from build123d import *

# Parameters (mm, degrees)
BOSS_EXTRUDE3_DEPTH = 31.75
BOSS_EXTRUDE4_DEPTH = 25.4
SKETCH3_R           = 12.7
BOSS_EXTRUDE5_DEPTH = 76.2


with BuildPart() as part:
    # Sketch1 → Boss-Extrude3 (new body)
    with BuildSketch(Plane.XY):
        with BuildLine():
            Line((-30.208002872, 9.539170605), (-46.704713672, 0.008989394))
            Line((-46.704713672, 0.008989394), (-30.209378213, -9.523572129))
            ThreePointArc((-30.209378213, -9.523572129), (-28.303227656, -4.925697376), (-27.653051773, 0.008989394))
            ThreePointArc((-27.653051773, 0.008989394), (-28.302871676, 4.942348519), (-30.208002872, 9.539170605))
        make_face()
        with BuildLine():
            Line((-30.209378213, -9.523572129), (-46.704713672, 0.008989394))
            Line((-46.704713672, 0.008989394), (-30.208002872, 9.539170605))
            ThreePointArc((-30.208002872, 9.539170605), (-65.756375522, 0.010363935), (-30.209378213, -9.523572129))
        make_face()
        with BuildLine():
            ThreePointArc((65.756375572, 53.972753345), (41.773446789, 72.372990127), (30.211103799, 44.443403463))
            Line((30.211103799, 44.443403463), (46.706375572, 53.972753345))
            Line((46.706375572, 53.972753345), (46.706375572, 34.922753345))
            ThreePointArc((46.706375572, 34.922753345), (60.176759753, 40.502369163), (65.756375572, 53.972753345))
        make_face()
        with BuildLine():
            Line((46.706375572, 53.972753345), (30.211103799, 44.443403463))
            ThreePointArc((30.211103799, 44.443403463), (37.183550761, 37.473713748), (46.706375572, 34.922753345))
            Line((46.706375572, 34.922753345), (46.706375572, 53.972753345))
        make_face()
        with BuildLine():
            ThreePointArc((46.706375572, -34.922753345), (37.184741159, -37.473026737), (30.21247902, -44.441023358))
            Line((30.21247902, -44.441023358), (46.706375572, -53.972753345))
            Line((46.706375572, -53.972753345), (46.706375572, -34.922753345))
        make_face()
        with BuildLine():
            Line((46.706375572, -53.972753345), (30.21247902, -44.441023358))
            ThreePointArc((30.21247902, -44.441023358), (41.772119261, -72.372634177), (65.756375572, -53.972753345))
            ThreePointArc((65.756375572, -53.972753345), (60.176759753, -40.502369163), (46.706375572, -34.922753345))
            Line((46.706375572, -34.922753345), (46.706375572, -53.972753345))
        make_face()
    extrude(amount=-BOSS_EXTRUDE3_DEPTH)

    # Sketch1_6 → Boss-Extrude4 (add)
    with BuildSketch(Plane.XY):
        Polygon((-46.704713672, 0.008989394), (46.706375572, -53.972753345), (46.706375572, 53.972753345), align=None)
    extrude(amount=BOSS_EXTRUDE4_DEPTH)

    # Sketch3 → Boss-Extrude5 (add)
    with BuildSketch(Plane.XY.offset(25.4)):
        with Locations(Location((15.593508684, 0, 0), (0, 0, 180))):
            Circle(SKETCH3_R)
    extrude(amount=BOSS_EXTRUDE5_DEPTH)


solid = part.part
Here's how the part is built. I have some questions about the finished solid (model axes, mm). A direction names the side the tool comes from. Give positions to 0.01 mm unless a question says otherwise; leave off trailing zeros. Write each loop counter-clockwise with the first axis right and the second up, starting at its lowest first coordinate (ties: lowest second). Pieces come first, ordered by that corner, then holes. Notation, with made-up numbers: (67, 47.5) -> (108, 47.5) arc R21 ccw to (108, 58.5) -> close; hole circle Ø9 at (61.5, 9.25). An arc over 180 degrees is marked (long way). Use one line per item in the form item = value. Start each with the question number.
1. Imagine slicing it at A-A on z = -2.5. List the corners of the cut face in (x, y) for me.
2. Imagine slicing it at B-B on y = -16. List the corners of the cut face in (x, z) for me.
3. Thinking about a two-plate mould opening in Y: for faces 1 (the face through (3.48, -3.81, 62.97)), 2 (the face through (46.706, -1, 13)), 3 (the face through (16, 1, 0)), 4 (the face through (-0.653, -26.604, 12.522)), which applies, +Y half, -Y half, draft (parallel to the pull), parting line (faces both ways), or undercut?
4. On a 3-axis mill with a long thin cutter (end or side, diameter ignored), from which of +Z, -Z, +X, -X, +Y, -Y can I reach the whole of each face in a straight line? I mean faces 5 (the face through (46, -54, -31.75)), 6 (the face through (0.655, 27.369, 12.522)), 7 (the face through (-48, 0, 0)). Say none if no direction works.
5. Imagine slicing it at C-C on x = 56. List the corners of the cut face in (y, z) for me.
6. If I drill on L1, parallel to Z at x = -11.5, y = 12; L2, parallel to Z at x = 48, y = 66; L3, parallel to X at y = -9, z = 35, over which ranges is the centre line in solid material (lowest first)?
7. Will these pins go through, and if not, where does the flat tip stop? pin 1 Ø20.5 at (y, z) = (9.5, 8) entering from +X; pin 2 Ø8 at (x, y) = (6.5, 18.5) entering from -Z; pin 3 Ø1 at (y, z) = (-16.5, -8) entering from -X.
8. Imagine slicing it at D-D on x = -38.5. List the corners of the cut face in (y, z) for me.
Entries:
q1.outline = circle Ø38.1 at (-46.7, 0.01); circle Ø38.1 at (46.71, -53.97); circle Ø38.1 at (46.71, 53.97)
q2.outline = (-57.03, -31.75) -> (-36.38, -31.75) -> (-36.38, 0) -> (-57.03, 0) -> close; (-19, 0) -> (46.71, 0) -> (46.71, 25.4) -> (-19, 25.4) -> close
q3.face_1 = parting line
q3.face_2 = draft
q3.face_3 = undercut
q3.face_4 = -Y half
q4.face_5 = -Z, +X, -X, +Y, -Y
q4.face_6 = +Z, -X, +Y
q4.face_7 = +Z, -X
q5.outline = (-70.6, -31.75) -> (-37.34, -31.75) -> (-37.34, 0) -> (-70.6, 0) -> close; (37.34, -31.75) -> (70.6, -31.75) -> (70.6, 0) -> (37.34, 0) -> close
q6.L1 = 0 to 25.4
q6.L2 = -31.75 to 0
q6.L3 = 6.63 to 24.55
q7.pin_1 = 46.71
q7.pin_2 = 0
q7.pin_3 = -57.03
q8.outline = (-17.19, -31.75) -> (17.2, -31.75) -> (17.2, 0) -> (4.75, 0) -> (4.75, 25.4) -> (-4.73, 25.4) -> (-4.73, 0) -> (-17.19, 0) -> close
